Part print with two shaded views. Sizes in mm from the minimum x, y, z corner. A direction names the side the tool comes from. Round coordinates to 2 decimals unless told otherwise and drop trailing zeros. Write each loop counter-clockwise with the first axis right and the second up, starting at its lowest first coordinate (ties: lowest second). Pieces come first, ordered by that corner, then holes. Notation, with made-up numbers: (12, 71) - (27, 71) arc R29 cw to (27, 100) - close; hole circle Ø1 at (13.25, 70.25). An arc over 180 degrees is marked (long way). Use one line per item in the form item = value. Start each with the question number.
Item 1: Pull direction Z, two halves, no side cores. Call the marked faces 1, 2 and 3: +Z half, -Z half, draft (parallel to the pull), parting line (faces both ways), or undercut.
Item 2: Band-saw the part on C-C, the plane z = 6.25. Give the number of separate pieces and of enclosed holes in the cut face.
Item 3: Drill centre lines: L1, parallel to Z at x = 7.5, y = 12.75; L2, parallel to Z at x = 5.5, y = 7.7; L3, parallel to Y at x = 5.25, z = 4.75 (1 decimal). Where is each one in solid material? Low to high.
Item 4: Tool access for the marked faces 4, 5 and 6: list every direction of +Z, -Z, +X, -X, +Y, -Y with a clear straight run to the whole face (end or side of a thin tool).
Item 5: Pin check, flat tips, straight feed: pin 1 (2.5 mm diameter, centred on x = 4, y = 13.5, fed in from -Z); pin 2 (1 mm diameter, centred on y = 2.5, z = 1, fed in from -X); pin 3 (3 mm diameter, centred on x = 1, y = 10.5, fed in from -Z); pin 4 (2 mm diameter, centred on y = 15, z = 3, fed in from +X). Stop position of each tip, or through.
Item 6: Band-saw the part on B-B, the plane y = 7.7. List the corners of the cut face in (x, z).
Item 7: Band-saw the part on D-D, the plane x = 4.5. List the corners of the cut face in (y, z) (1 decimal).
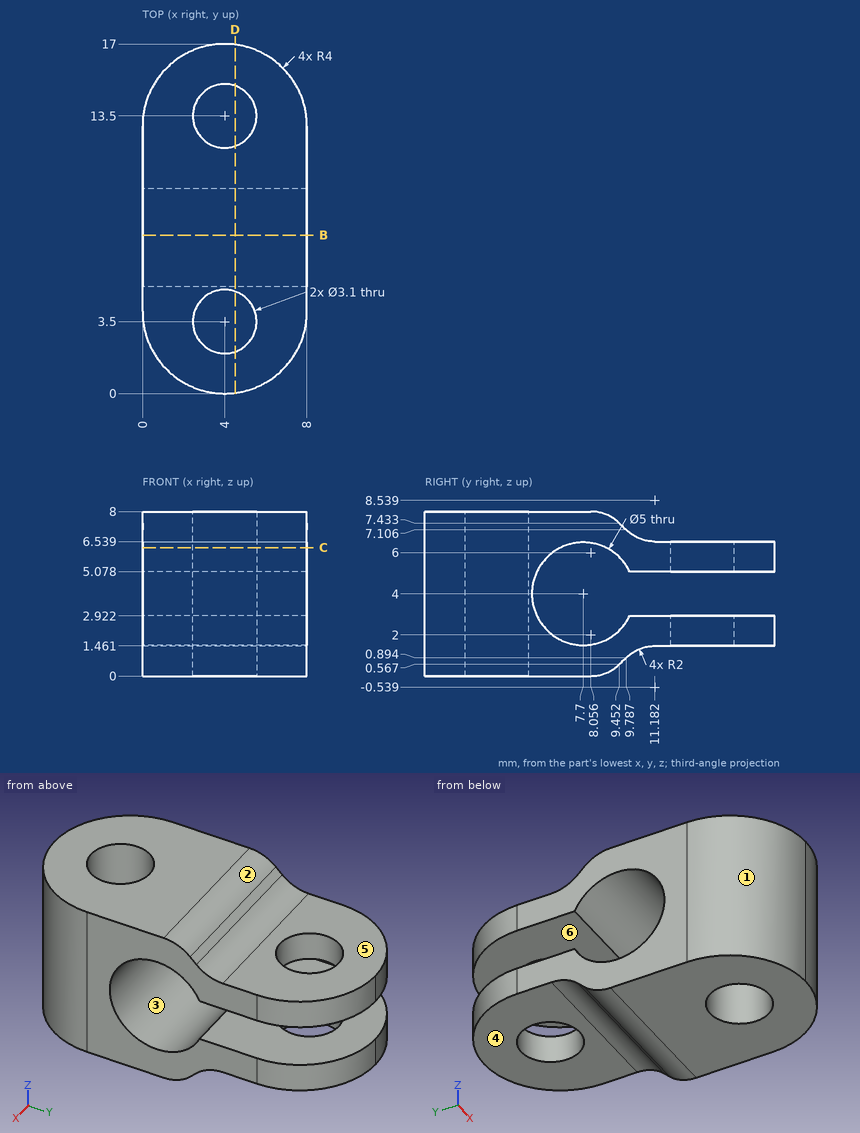
Determined:
q1.face_1 = draft
q1.face_2 = +Z half
q1.face_3 = undercut
q2.separate_pieces = 2
q2.enclosed_holes = 2
q3.L1 = 1.46 to 2.92, 5.08 to 6.54
q3.L2 = 0 to 1.5, 6.5 to 8
q3.L3 = 0.2 to 2.6, 4.4 to 5.3
q4.face_4 = -Z, +X, -X, +Y
q4.face_5 = +Z, +X, -X, +Y
q4.face_6 = +X, -X, +Y
q5.pin_1 = through
q5.pin_2 = 0.13
q5.pin_3 = 0.24
q5.pin_4 = 7.87
q6.outline = (0, 0) - (8, 0) - (8, 1.5) - (0, 1.5) - close; (0, 6.5) - (8, 6.5) - (8, 8) - (0, 8) - close
q7.outline = (0, 0) - (2, 0) - (2, 8) - (0, 8) - close; (5, 0) - (8.1, 0) arc R2 ccw to (9.5, 0.6) - (9.8, 0.9) arc R2 cw to (11.2, 1.5) - (12, 1.5) - (12, 2.9) - (10, 2.9) arc R2.5 cw (long way) to (10, 5.1) - (12, 5.1) - (12, 6.5) - (11.2, 6.5) arc R2 cw to (9.8, 7.1) - (9.5, 7.4) arc R2 ccw to (8.1, 8) - (5, 8) - close; (15, 1.5) - (17, 1.5) - (17, 2.9) - (15, 2.9) - close; (15, 5.1) - (17, 5.1) - (17, 6.5) - (15, 6.5) - close
